Geometry: final body of the model. Coordinates: model frame, mm. Coordinates: 2 decimals unless noted, no trailing zeros. Write each loop counter-clockwise with the first axis right and the second up, starting at its lowest first coordinate (ties: lowest second). Pieces come first, ordered by that corner, then holes. Notation, with made-up numbers: (54.25, -26) -> (83.25, -26) arc R14 ccw to (83.25, 1) -> close; hole circle Ø10 at (22.5, -22). An arc over 180 degrees is marked (long way). One line per item, written item: value.
```python
from build123d import *

# Parameters (mm, degrees)
SKETCH1_R           = 2.38125
SKETCH1_R_2         = 14.2875
SKETCH1_R_3         = 8.75
BOSS_EXTRUDE1_DEPTH = 6.35
SKETCH2_R           = 2.54
CUT_EXTRUDE1_DEPTH  = 6.35


with BuildPart() as part:
    # Sketch1 → Boss-Extrude1 (new body)
    with BuildSketch(Plane.XY):
        with BuildLine():
            Line((-25.4, 27.94), (38.1, 27.94))
            ThreePointArc((38.1, 27.94), (42.590128061, 26.080128061), (44.45, 21.59))
            Line((44.45, 21.59), (44.45, -67.31))
            ThreePointArc((44.45, -67.31), (42.590128061, -71.800128061), (38.1, -73.66))
            Line((38.1, -73.66), (-25.4, -73.66))
            ThreePointArc((-25.4, -73.66), (-29.890128061, -71.800128061), (-31.75, -67.31))
            Line((-31.75, -67.31), (-31.75, 21.59))
            ThreePointArc((-31.75, 21.59), (-29.890128061, 26.080128061), (-25.4, 27.94))
        make_face()
        with Locations((14.5, 0)):
            Circle(SKETCH1_R, mode=Mode.SUBTRACT)
        with Locations((-14.5, 0)):
            Circle(SKETCH1_R, mode=Mode.SUBTRACT)
        with Locations((14.5, -45.72)):
            Circle(SKETCH1_R, mode=Mode.SUBTRACT)
        with Locations((-14.5, -45.72)):
            Circle(SKETCH1_R, mode=Mode.SUBTRACT)
        with Locations((19.677317049, -22.86)):
            Circle(SKETCH1_R_2, mode=Mode.SUBTRACT)
        with Locations((0, -45.72)):
            Circle(SKETCH1_R_3, mode=Mode.SUBTRACT)
        Circle(SKETCH1_R_3, mode=Mode.SUBTRACT)
    extrude(amount=BOSS_EXTRUDE1_DEPTH)

    # Sketch2 → Cut-Extrude1 (cut)
    with BuildSketch(Plane.XY.offset(6.35)):
        with Locations((-22.225, 15.24)):
            Circle(SKETCH2_R)
        with Locations((31.75, 15.24)):
            Circle(SKETCH2_R)
        with Locations((31.75, -60.96)):
            Circle(SKETCH2_R)
        with Locations((-22.225, -60.96)):
            Circle(SKETCH2_R)
    extrude(amount=-CUT_EXTRUDE1_DEPTH, mode=Mode.SUBTRACT)


solid = part.part
```
(1) Pull-direction query (X, two-part tool) for faces 1 (the flat face through (6, 27.94, 3)), 2 (the cylindrical face through (-1.139, -37.044, 3.131)), 3 (the flat face through (-31.75, -23, 3)), 4 (the flat face through (44.45, -22, 3)); classes: released by +X, released by -X, zero draft, split by the parting line, or undercut.
Responses:
face 1: zero draft
face 2: undercut
face 3: released by -X
face 4: released by +X
(2) Section A-A (x = 0). Return the cut outline in (y, z), then the cut area to 3 significant figures.
Responses:
outline: (-73.66, 0) -> (-54.47, 0) -> (-54.47, 6.35) -> (-73.66, 6.35) -> close; (-36.97, 0) -> (-8.75, 0) -> (-8.75, 6.35) -> (-36.97, 6.35) -> close; (8.75, 0) -> (27.94, 0) -> (27.94, 6.35) -> (8.75, 6.35) -> close
area: 423 mm2
(3) Section B-B (y = -60.96). Return the cut outline in (x, z) (3 decimals).
Responses:
outline: (-31.75, 0) -> (-24.765, 0) -> (-24.765, 6.35) -> (-31.75, 6.35) -> close; (-19.685, 0) -> (29.21, 0) -> (29.21, 6.35) -> (-19.685, 6.35) -> close; (34.29, 0) -> (44.45, 0) -> (44.45, 6.35) -> (34.29, 6.35) -> close
(4) Section C-C (y = -45.72). Return the cut outline in (x, z).
Responses:
outline: (-31.75, 0) -> (-16.88, 0) -> (-16.88, 6.35) -> (-31.75, 6.35) -> close; (-12.12, 0) -> (-8.75, 0) -> (-8.75, 6.35) -> (-12.12, 6.35) -> close; (8.75, 0) -> (12.12, 0) -> (12.12, 6.35) -> (8.75, 6.35) -> close; (16.88, 0) -> (44.45, 0) -> (44.45, 6.35) -> (16.88, 6.35) -> close
(5) Line query: line 1 (Y direction, x = -14.5, z = 2.75); line 2 (Y direction, x = 0, z = 4); line 3 (X direction, y = 15, z = 3). Output: solid intervals per line, ascending. Write a range as [from, to].
Responses:
line 1: y = [-73.66, -48.1], [-43.34, -2.38], [2.38, 27.94]
line 2: y = [-73.66, -54.47], [-36.97, -8.75], [8.75, 27.94]
line 3: x = [-31.75, -24.75], [-19.7, 29.22], [34.28, 44.45]
(6) Section D-D (z = 1.75). State how many separate pieces and enclosed holes the cut face has, then the cut area to 3 significant figures.
Responses:
separate pieces: 1
enclosed holes: 11
area: 6,430 mm2
